For this review, use the dimensioned drawing (mm, ordinates from the lowest corner) and the shaded views. A direction names the side the tool comes from. Round coordinates to 2 decimals unless told otherwise and drop trailing zeros. Write each loop counter-clockwise with the first axis right and the second up, starting at its lowest first coordinate (ties: lowest second). Pieces come first, ordered by that corner, then holes. Notation, with made-up numbers: M 62.5,29.5 L 90.5,29.5 A16 ccw 90.5,56.5 Z; hole C 35,74.25 d11. An arc over 180 degrees is marked long. Answer in a Markdown table with one row per item.
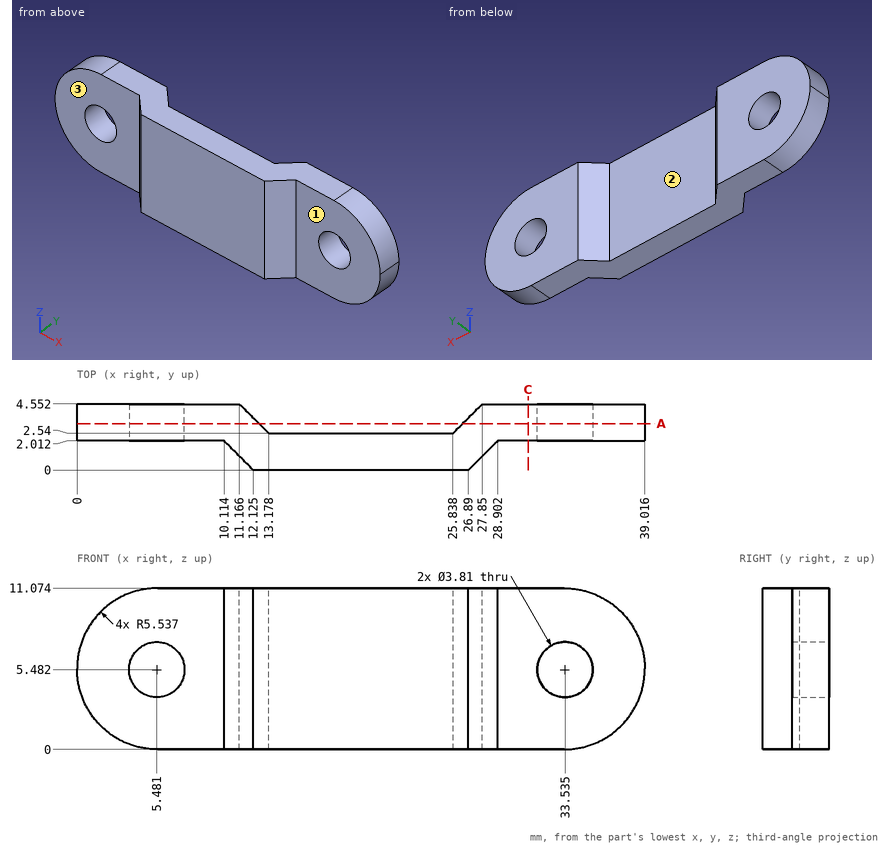
Q1. Machinability: for the marked faces 1, 2 and 3, which of the approach directions +Z, -Z, +X, -X, +Y, -Y give a long, thin tool a straight path to every point of the face, cutting with its end or side? Answer none if there is none.
Found:
| item | result |
|---|---|
| face 1 | +Z, -Z, +X, -Y |
| face 2 | +Z, -Z, +Y |
| face 3 | +Z, -Z, -X, -Y |
Q2. For probe 1 along X at (y, z) = (2.5, 6) (1 decimal); probe 2 along X at (y, z) = (2.5, 4) (1 decimal); probe 3 along Y at (x, z) = (15.5, 3), list the stretches that pass through material, from the lowest coordinate up.
Found:
| item | result |
|---|---|
| probe 1 | 0 to 3.6, 7.3 to 31.7, 35.4 to 39 |
| probe 2 | 0.2 to 4.3, 6.7 to 32.3, 34.7 to 38.8 |
| probe 3 | 0 to 2.54 |
Q3. Insertion check: P1, Ø3, axis at x = 35.5, z = 5, coming from the -Y side; P2, Ø4, axis at x = 12, z = 9, coming from the -Y side; P3, Ø2, axis at y = 3, z = 7.5, coming from the -X side (1 decimal). Each pin has a flat end and moves straight along its axis. Give the tip position at first contact, or say it passes through.
Found:
| item | result |
|---|---|
| P1 | y = 2.01 |
| P2 | y = 0 |
| P3 | x = 0.1 |
Q4. Take a section at C-C (x = 31). State the section outline as (y, z) points (1 decimal).
Found:
| item | result |
|---|---|
| outline | M 2,0 L 4.6,0 L 4.6,11.1 L 2,11.1 Z |
Q5. Take a section at A-A (y = 3.2). State how many separate pieces and enclosed holes the cut face has, then the cut area to 3 significant figures.
Found:
| item | result |
|---|---|
| separate pieces | 2 |
| enclosed holes | 2 |
| area | 228 mm² |
